Can you work these out from the model? Positions are in its coordinate system, mm. A direction names the side the tool comes from. Round coordinates to 2 decimals unless told otherwise and drop trailing zeros. Loops run counter-clockwise (first coordinate to the right, second up) from the corner with the lowest first, then second, coordinate; pieces in that order, holes last. Notation, with made-up numbers: M 41,4.25 L 91,4.25 A29 ccw 91,34.25 Z; hole C 12,82.25 d10. An arc over 180 degrees is marked long. Use a Markdown table: item, result. Add a question column.
```python
from build123d import *

# Parameters (mm, degrees)
SKETCH2_R                              = 14
BOSS_EXTRUDE1_DEPTH                    = 3
SKETCH3_R                              = 6
BOSS_EXTRUDE2_DEPTH                    = 26.5
BOSS_EXTRUDE3_DEPTH                    = 1
BOSS_EXTRUDE4_REACH                    = 80.443
BOSS_EXTRUDE4_END_RADIUS               = 6
M36_CLEARANCE_HOLE1_D                  = 39
M36_CLEARANCE_HOLE1_DEPTH              = 4.45
F_1_5_1_5_DIAMETER_HOLE1_D             = 1.5
F_1_5_1_5_DIAMETER_HOLE1_DEPTH         = 2
F_1_5_1_5_DIAMETER_HOLE1_TIP           = 0.450645464
F_3_3_3_3_DIAMETER_HOLE1_D             = 3.3
F_3_3_3_3_DIAMETER_HOLE1_DEPTH         = 6
F_3_3_3_3_DIAMETER_HOLE1_TIP           = 0.991420021
F_1_25_1_25_DIAMETER_HOLE1_D           = 1.25
F_1_25_1_25_DIAMETER_HOLE1_DEPTH       = 1.939156082
F_1_25_1_25_DIAMETER_HOLE1_CSINK_D     = 2.65
F_1_25_1_25_DIAMETER_HOLE1_CSINK_ANGLE = 60
F_1_25_1_25_DIAMETER_HOLE1_TIP         = 0.360843918
CHAMFER1_SIZE                          = 0.288675135
CHAMFER1_SIZE2                         = 0.5


with BuildPart() as part:
    # Sketch1 → Revolve1 (revolve)
    with BuildSketch(Plane.XY, mode=Mode.PRIVATE) as revolve1_sk:
        with BuildLine():
            Line((0, 21), (0, 0))
            Line((0, 0), (70, 0))
            Line((70, 0), (70, 21))
            Line((70, 21), (9.25, 21))
            ThreePointArc((9.25, 21), (9.2, 20.98660254), (9.15, 21))
            Line((9.15, 21), (0, 21))
        make_face()
    revolve(revolve1_sk.sketch.rotate(Axis((0, 0, 0), (1, 0, 0)), 270), axis=Axis((0, 0, 0), (1, 0, 0)))

    # Sketch2 → Boss-Extrude1 (add)
    with BuildSketch(Plane.ZY):
        Circle(SKETCH2_R)
    extrude(amount=BOSS_EXTRUDE1_DEPTH)

    # Sketch3 → Boss-Extrude2 (add)
    with BuildSketch(Plane.ZY.offset(3)):
        Circle(SKETCH3_R)
    extrude(amount=BOSS_EXTRUDE2_DEPTH)

    # Sketch4 → Boss-Extrude3 (add)
    with BuildSketch(Plane.ZY.offset(3)):
        with BuildLine():
            Line((0.293916284, -7.616838781), (0.293916284, -5.992796778))
            ThreePointArc((0.293916284, -5.992796778), (0, 6), (-0.293916284, -5.992796778))
            Line((-0.293916284, -5.992796778), (-0.293916284, -7.616838781))
            ThreePointArc((-0.293916284, -7.616838781), (-1.755912185, -7.072113956), (-2.882513969, -5.992796778))
            ThreePointArc((-2.882513969, -5.992796778), (0, 6.65), (2.882513969, -5.992796778))
            ThreePointArc((2.882513969, -5.992796778), (1.821852016, -7.17721696), (0.293916284, -7.616838781))
        make_face()
    extrude(amount=BOSS_EXTRUDE3_DEPTH)

    # Boss-Extrude4: up to this cylinder (the profile starts outside it)
    boss_extrude4_end = Plane(origin=(-17.5, 0, 0), z_dir=(1, 0, 0)) * Cylinder(BOSS_EXTRUDE4_END_RADIUS, 173.886, mode=Mode.PRIVATE)
    # Sketch5 → Boss-Extrude4 (add, up to the surface)
    with BuildSketch(Plane(origin=(0, 7.5, 0), x_dir=(1, 0, 0), z_dir=(0, 1, 0)), mode=Mode.PRIVATE) as boss_extrude4_sk1:
        with BuildLine():
            Line((-9.5, 2), (-25.5, 2))
            ThreePointArc((-25.5, 2), (-27.5, 0), (-25.5, -2))
            Line((-25.5, -2), (-9.5, -2))
            ThreePointArc((-9.5, -2), (-7.5, 0), (-9.5, 2))
        make_face()
    boss_extrude4_tool1 = extrude(boss_extrude4_sk1.sketch, amount=-BOSS_EXTRUDE4_REACH, mode=Mode.PRIVATE) - boss_extrude4_end
    add(boss_extrude4_tool1.solids().sort_by_distance((-17.5, 7.5, 0))[0])

    # M36 Clearance Hole1
    with Locations(Plane(origin=(70, 0, 0), x_dir=(0, 0, -1), z_dir=(1, 0, 0))):
        with Locations((0, 0)):
            Hole(M36_CLEARANCE_HOLE1_D / 2, depth=M36_CLEARANCE_HOLE1_DEPTH)

    # Ø1.5 (1.5) Diameter Hole1
    with Locations(Plane.ZY):
        with Locations((-7.462326931, 18.015650884)):
            Hole(F_1_5_1_5_DIAMETER_HOLE1_D / 2, depth=F_1_5_1_5_DIAMETER_HOLE1_DEPTH)
            with Locations((0, 0, -(F_1_5_1_5_DIAMETER_HOLE1_DEPTH + F_1_5_1_5_DIAMETER_HOLE1_TIP / 2))):  # 118° drill point
                Cone(0, F_1_5_1_5_DIAMETER_HOLE1_D / 2, F_1_5_1_5_DIAMETER_HOLE1_TIP, mode=Mode.SUBTRACT)

    # Ø3.3 (3.3) Diameter Hole1
    with Locations(Plane.ZY):
        with Locations((3.0543e-05, 17.5), (17.5, -3.0543e-05), (-3.0543e-05, -17.5), (-17.5, 3.0543e-05)):
            Hole(F_3_3_3_3_DIAMETER_HOLE1_D / 2, depth=F_3_3_3_3_DIAMETER_HOLE1_DEPTH)
            with Locations((0, 0, -(F_3_3_3_3_DIAMETER_HOLE1_DEPTH + F_3_3_3_3_DIAMETER_HOLE1_TIP / 2))):  # 118° drill point
                Cone(0, F_3_3_3_3_DIAMETER_HOLE1_D / 2, F_3_3_3_3_DIAMETER_HOLE1_TIP, mode=Mode.SUBTRACT)

    # Ø1.25 (1.25) Diameter Hole1
    with Locations(Plane.ZY.offset(29.5)):
        with Locations((0, 0)):
            CounterSinkHole(F_1_25_1_25_DIAMETER_HOLE1_D / 2, F_1_25_1_25_DIAMETER_HOLE1_CSINK_D / 2, depth=F_1_25_1_25_DIAMETER_HOLE1_DEPTH, counter_sink_angle=F_1_25_1_25_DIAMETER_HOLE1_CSINK_ANGLE)
            with Locations((0, 0, -(F_1_25_1_25_DIAMETER_HOLE1_DEPTH + F_1_25_1_25_DIAMETER_HOLE1_TIP / 2))):  # 120° drill point
                Cone(0, F_1_25_1_25_DIAMETER_HOLE1_D / 2, F_1_25_1_25_DIAMETER_HOLE1_TIP, mode=Mode.SUBTRACT)

    # Chamfer1
    chamfer1_edges = [part.edges().sort_by_distance(p)[0] for p in [
        (-29.5, 0, -6),
    ]]
    chamfer1_side = [part.faces().sort_by_distance(p)[0] for p in [
        (-29.5, 0, -5.830294373),
    ]]
    chamfer(chamfer1_edges, length=CHAMFER1_SIZE, length2=CHAMFER1_SIZE2, reference=chamfer1_side[0])


solid = part.part
```
(1) Thinking about a two-plate mould opening in Y: for faces 4 (the face through (39.2, 6.31, -20.03)), 5 (the face through (3.04, 18.89, -0.89)), 6 (the face through (67.744, 19.334, -2.539)), 7 (the face through (-3, -6, -3.3)), which applies, released by +Y, released by -Y, zero draft, split by the parting line, or undercut?
(2) Suppose I cut it at A-A on x = -20.5. List the corners of the cut face in (y, z) for me, and give its area (3 significant figures).
(3) On a 3-axis mill with a long thin cutter (end or side, diameter ignored), from which of +Z, -Z, +X, -X, +Y, -Y can I reach the whole of each face in a straight line? I mean faces 1 (the face through (3.04, -16.11, -0.89)), 2 (the face through (-18, 7, 2)), 3 (the face through (-18, 7.5, 0)). Say none if no direction works.
(4) I'm going to push flat-ended pins straight in: pin 1 (1.6 mm diameter, centred on y = 0, z = 0, fed in from +X); pin 2 (1.5 mm diameter, centred on x = -16, y = 7, fed in from +Z); pin 3 (1 mm diameter, centred on x = 58, z = -14, fed in from +Y). Where does each tip first touch, or does it pass through?
(5) If I drill on probe 1 along X at (y, z) = (-9, 15.5); probe 2 along X at (y, z) = (-1, -6); probe 3 along Y at (x, z) = (67.4, 0), over which ranges is the centre line in solid material (lowest first)? Write a range as [from, to].
Results below:
| question | item | result |
|---|---|---|
| 1 | face 4 | split by the parting line |
| 1 | face 5 | undercut |
| 1 | face 6 | undercut |
| 1 | face 7 | zero draft |
| 2 | outline | M 5.66,-2 L 7.5,-2 L 7.5,2 L 5.66,2 A6 ccw long Z |
| 2 | area | 120 mm² |
| 3 | face 1 | -X |
| 3 | face 2 | +Z, -X, +Y |
| 3 | face 3 | +Z, -Z, -X, +Y |
| 4 | pin 1 | stops at x = 65.55 |
| 4 | pin 2 | stops at z = 2 |
| 4 | pin 3 | stops at y = 16.09 |
| 5 | probe 1 | x = [0, 65.55] |
| 5 | probe 2 | x = [-4, 65.55] |
| 5 | probe 3 | y = [-21, -19.5], [19.5, 21] |
